Geometry check sheet. Reference: drawing and pictorial views, mm from the part's lowest x, y, z. A direction names the side the tool comes from. Give positions to 0.01 mm unless a question says otherwise; leave off trailing zeros. Order: outer loops, then holes, each group sorted by start corner. A loop starts at its lowest first (then second) coordinate and runs counter-clockwise, first axis right, second up.
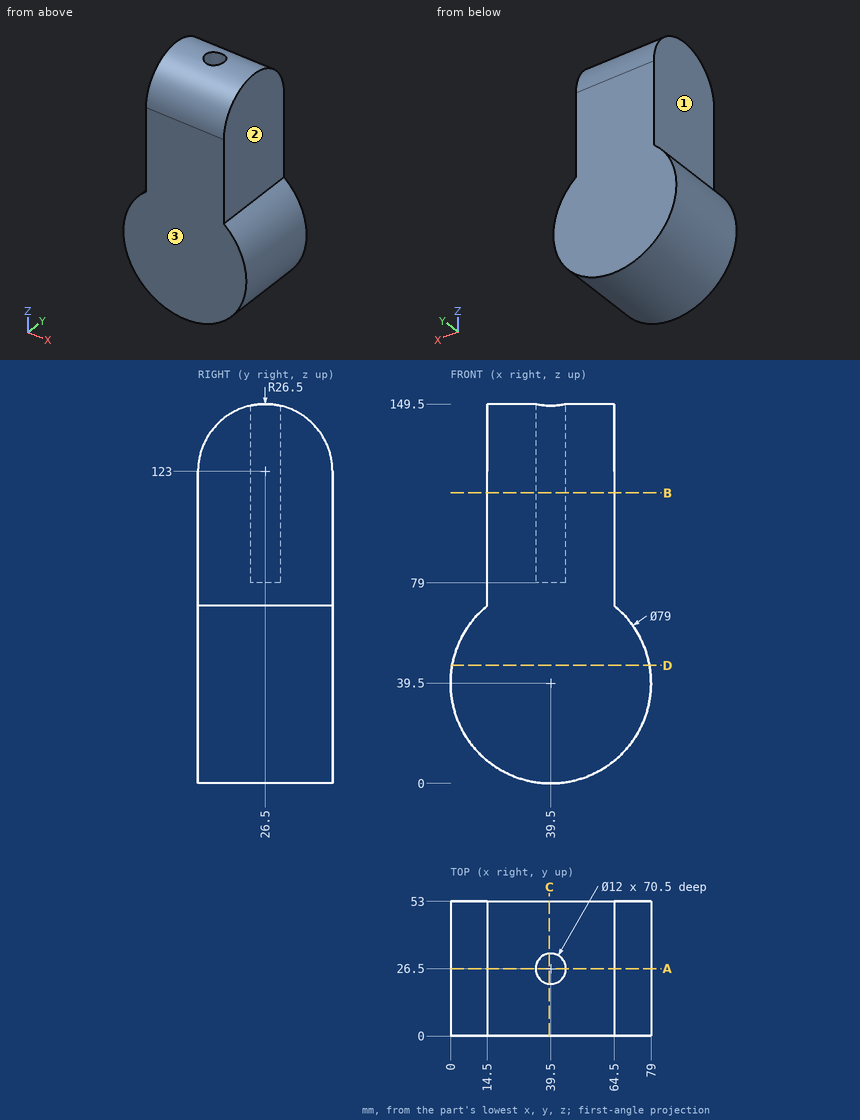
(1) Cross-section at B-B on z = 114.5. Enter the section's corners in (x, y), then the cut area to 3 significant figures.
Response values:
outline: (14.5, 0) - (64.5, 0) - (64.5, 53) - (14.5, 53) - close; hole circle Ø12 at (39.5, 26.5)
area: 2,540 mm2
(2) Material ranges on L1, parallel to X at y = 26, z = 111; L2, parallel to X at y = 35, z = 107; L3, parallel to Y at x = 39.5, z = 96, recorded low to high.
Response values:
L1: x = 14.5 to 33.52, 45.48 to 64.5
L2: x = 14.5 to 64.5
L3: y = 0 to 20.5, 32.5 to 53
(3) Set-up check for the marked faces 1, 2 and 3: record each of +Z, -Z, +X, -X, +Y, -Y from which the full face is reachable in a straight line by a thin tool's end or side.
Response values:
face 1: +Z, -X, +Y, -Y
face 2: +Z, +X, +Y, -Y
face 3: +Z, -Z, +X, -X, -Y
(4) Cross-section at D-D on z = 46.5. Enter the section's corners in (x, y), then the cut area to 3 significant figures.
Response values:
outline: (0.63, 0) - (78.37, 0) - (78.37, 53) - (0.63, 53) - close
area: 4,120 mm2
(5) Gauge pin test, flat ends, axial feed: pin 1 Ø4 at (y, z) = (8, 39) entering from -X; pin 2 Ø12 at (x, y) = (44.5, 24) entering from +Z; pin 3 Ø9.5 at (x, y) = (40, 24.5) entering from +Z; pin 4 Ø3 at (x, y) = (69, 22.5) entering from +Z. Record the tip position at first contact, or that the pin passes through.
Response values:
pin 1: stops at x = 0
pin 2: stops at z = 149.5
pin 3: stops at z = 149.31
pin 4: stops at z = 67.36
(6) Cross-section at A-A on y = 26.5. Enter the section's corners in (x, z).
Response values:
outline: (14.5, 70.08) arc R39.5 ccw (long way) to (64.5, 70.08) - (64.5, 149.5) - (45.5, 149.5) - (45.5, 79) - (33.5, 79) - (33.5, 149.5) - (14.5, 149.5) - close
(7) Cross-section at C-C on x = 39. Enter the section's corners in (y, z).
Response values:
outline: (0, 0) - (53, 0) - (53, 123) arc R26.5 ccw to (32.48, 148.82) - (32.48, 79) - (20.52, 79) - (20.52, 148.82) arc R26.5 ccw to (0, 123) - close
